Solid Edge part; units mm, degrees
sketch "Sketch1" plane through (0, 0, 0) normal (0, -1, 0) x (1, 0, 0)
  line L0 (2.5, 0) -> (2.5, 5)
  line L1 (2.5, 5) -> (2.4, 5.1)
  line L2 (2.4, 5.1) -> (2.4, 10)
  line L3 (2.4, 10) -> (0, 10)
  line L4 (2.5, 0) -> (0, 0)
  dimension "D1" = 2.5
revolve "RevolvedProtrusion1" add sketch "Sketch1" angle 360 about axis through (0, 0, 0) along (0, 0, 1)
sketch "Sketch2" plane through (0, 0, 0) normal (0, 0, -1) x (-1, 0, 0)
  line L0 (-0.7217, 1.25) -> (-1.4434, 0)
  line L1 (-1.4434, 0) -> (-0.7217, -1.25)
  line L2 (-0.7217, -1.25) -> (0.7217, -1.25)
  line L3 (0.7217, -1.25) -> (1.4434, 0)
  line L4 (1.4434, 0) -> (0.7217, 1.25)
  line L5 (0.7217, 1.25) -> (-0.7217, 1.25)
extrude "Cutout1" cut sketch "Sketch2" along normal mid plane 6
chamfer "Chamfer_1" distance 0.5 angle 45 1 edges at (-2.4, 0, 10)
cosmetic_thread "Thread1"
properties material "Steel"
Verification items for the finished model (mm, model axes). A direction names the side the tool comes from. Coordinates: 2 decimals unless noted, no trailing zeros. Order: outer loops, then holes, each group sorted by start corner. A loop starts at its lowest first (then second) coordinate and runs counter-clockwise, first axis right, second up. Notation, with made-up numbers: M -34.5,-38.75 L -15.5,-38.75 A27 ccw -15.5,0.25 Z; hole C -24.75,69 d10. An arc over 180 degrees is marked long. One line per item, written item: value. Start each with the question number.
Item 1: Depth check by flat-ended pin: P1, Ø2, axis at y = -1.5, z = 6.5, coming from the -X side; P2, Ø0.8, axis at x = 0.5, y = 0.5, coming from the -Z side. Enter the tip coordinate at first touch or a pass-through.
Item 2: Sectioned sample at B-B on x = 0. Record the cut outline in (y, z), then the cut area to 3 significant figures.
Item 3: Thickness scan on probe 1 along Y at (x, z) = (-0.85, 0.5); probe 2 along Z at (x, y) = (0.75, -1.05); probe 3 along X at (y, z) = (0.55, 1.75). Record the ranges inside material, lowest first.
Item 4: Access from +Z, -Z, +X, -X, +Y, -Y to the whole of each face (thin tool, end or side, straight path). Record for faces 1 (the cylindrical face through (1.29, 2.024, 7.331)), 2 (the flat face through (0, 0, 10)), 3 (the flat face through (1.088, -0.616, 1.521)).
Item 5: Sectioned sample at C-C on z = 6. Record the cut outline in (x, y), then the cut area to 3 significant figures.
Item 6: Sectioned sample at A-A on z = 2.75. Record the cut outline in (x, y).
Item 7: Sectioned sample at D-D on z = 4.25. Record the cut outline in (x, y).
Item 8: Mould release check, pull along Y, two halves, no side actions. Record for faces 4 (the flat face through (1.1, -1.1, 0)), 5 (the cylindrical face through (-0.54, -2.44, 2.54)), 6 (the flat face through (0, -1.25, 2)): pulls with the +Y half, pulls with the -Y half, needs draft (parallel to the pull), parting line crosses it, or undercut.
Calculated:
1. P1: x = -2.35
1. P2: z = 3
2. outline: M -2.5,0 L -1.25,0 L -1.25,3 L 1.25,3 L 1.25,0 L 2.5,0 L 2.5,5 L 2.4,5.1 L 2.4,9.5 L 1.9,10 L -1.9,10 L -2.4,9.5 L -2.4,5.1 L -2.5,5 Z
2. area: 41.3 mm^2
3. probe 1: -2.35 to -1.03, 1.03 to 2.35
3. probe 2: 3 to 10
3. probe 3: -2.44 to -1.13, 1.13 to 2.44
4. face 1: +Z
4. face 2: +Z, +X, -X, +Y, -Y
4. face 3: -Z
5. outline: C 0,0 d4.8
5. area: 18.1 mm^2
6. outline: C 0,0 d5; hole M -1.44,0 L -0.72,-1.25 L 0.72,-1.25 L 1.44,0 L 0.72,1.25 L -0.72,1.25 Z
7. outline: C 0,0 d5
8. face 4: needs draft
8. face 5: parting line crosses it
8. face 6: undercut
